The listing builds one solid part. Answer for the finished solid, in the listing's coordinates (mm). A direction names the side the tool comes from. Round coordinates to 2 decimals unless told otherwise and drop trailing zeros. Loops run counter-clockwise (first coordinate to the right, second up) from the corner with the lowest first, then second, coordinate; pieces in that order, holes last. Notation, with made-up numbers: M 82,42.25 L 119,42.25 A4 ccw 119,47.25 Z; hole C 84,42.5 d10. An arc over 180 degrees is marked long. Answer as a JSON object with one key per item and string values.
```python
from build123d import *

# Parameters (mm, degrees)
F0_W            = 25.4
F0_H            = 38.1
F1_DEPTH        = 12.7
F3_DEPTH        = 76.2
F4_W            = 25.4
F4_H            = 6.346226
F5_DEPTH        = 63.5
F7_DEPTH        = 25.4
F8_W            = 25.4
F8_H            = 6.35
F9_DEPTH        = 12.7
F11_DEPTH       = 25.4
F13_D           = 2.38125
F13_DEPTH       = 12.7
F13_CBORE_D     = 6.35
F13_CBORE_DEPTH = 3.175


with BuildPart() as f1:
    # F0 (on Front) → F1 (new body)
    with BuildSketch(Plane.XZ):
        with Locations((-20.66209, -15.939255)):
            Rectangle(F0_W, F0_H)
    extrude(amount=-F1_DEPTH)

    # F2 (on face) → F3 (join)
    with BuildSketch(Plane(origin=(0, 12.7, 0), x_dir=(-1, 0, 0), z_dir=(0, 1, 0))):
        Polygon((7.96209, -9.589255), (20.66209, -9.589255), (33.36209, -9.589255), (33.36209, 3.110745), (7.96209, 3.110745), align=None)
    extrude(amount=F3_DEPTH)

    # F4 (on face) → F5 (join)
    with BuildSketch(Plane(origin=(0, 0, -9.589255), x_dir=(1, 0, 0), z_dir=(0, 0, -1))):
        with Locations((-20.66209, -85.726887)):
            Rectangle(F4_W, F4_H)
    extrude(amount=F5_DEPTH)

    # F6 (on face) → F7 (join)
    with BuildSketch(Plane.YZ.offset(-7.96209)):
        Polygon((57.153774, -9.589255), (82.553774, -34.989255), (82.553774, -9.589255), align=None)
    extrude(amount=-F7_DEPTH)

    # F8 (on face) → F9 (join)
    with BuildSketch(Plane(origin=(0, 12.7, 0), x_dir=(-1, 0, 0), z_dir=(0, 1, 0))):
        with Locations((20.66209, -12.764255)):
            Rectangle(F8_W, F8_H)
    extrude(amount=F9_DEPTH)

    # F10 (on face) → F11 (cut, through all)
    with BuildSketch(Plane.YZ.offset(-7.96209)):
        Polygon((25.4, -15.939255), (25.4, -9.589255), (12.7, -15.939255), align=None)
    extrude(amount=-F11_DEPTH, mode=Mode.SUBTRACT)

    # F13
    with Locations(Plane(origin=(0, 12.7, 0), x_dir=(-1, 0, 0), z_dir=(0, 1, 0))):
        with Locations((20.66209, -25.464255)):
            CounterBoreHole(F13_D / 2, F13_CBORE_D / 2, F13_CBORE_DEPTH, depth=F13_DEPTH)


solid = f1.part
```
Item 1: Which of the six approach directions +Z, -Z, +X, -X, +Y, -Y give full straight-line access (tool end or side, diameter ignored) to faces 1 (the face through (-20, 41, -9.589)), 2 (the face through (-21, 82.554, -54)), 3 (the face through (-20.92, 4.696, -26.627))?
Values follow:
{"face 1": "-Z, +X, -X", "face 2": "-Z, +X, -X, -Y", "face 3": "-Y"}
Item 2: The part is cut by section D-D (y = 34). Give the vertices of the cut face in (x, z), then the cut area to 3 significant figures.
Values follow:
{"outline": "M -33.36,-9.59 L -7.96,-9.59 L -7.96,3.11 L -33.36,3.11 Z", "area": "323 mm^2"}
Item 3: The part is cut by section A-A (z = -14.5). Give the vertices of the cut face in (x, y), then the cut area to 3 significant figures.
Values follow:
{"outline": "M -33.36,0 L -7.96,0 L -7.96,15.58 L -33.36,15.58 Z; M -33.36,62.06 L -7.96,62.06 L -7.96,88.9 L -33.36,88.9 Z", "area": "1,080 mm^2"}
Item 4: The part is cut by section B-B (x = -12). Give the vertices of the cut face in (y, z).
Values follow:
{"outline": "M 0,-34.99 L 12.7,-34.99 L 12.7,-15.94 L 25.4,-9.59 L 57.15,-9.59 L 82.55,-34.99 L 82.55,-73.09 L 88.9,-73.09 L 88.9,3.11 L 0,3.11 Z"}
Item 5: The part is cut by section C-C (z = -67.5). Give the vertices of the cut face in (x, y), then the cut area to 3 significant figures.
Values follow:
{"outline": "M -33.36,82.55 L -7.96,82.55 L -7.96,88.9 L -33.36,88.9 Z", "area": "161 mm^2"}
Item 6: Straight lines are drawn through the part: line 1 (Y direction, x = -10.75, z = -46); line 2 (Y direction, x = -13, z = -17); line 3 (Y direction, x = -29.5, z = -13). For each, find the intervals that lie inside material, in ascending order.
Values follow:
{"line 1": "82.55 to 88.9", "line 2": "0 to 12.7, 64.56 to 88.9", "line 3": "0 to 18.58, 60.56 to 88.9"}
Item 7: Determine the mould class of faces 4 (the face through (-20.48, 19.14, -12.72)), 5 (the face through (-21, 44, 3.111)), 6 (the face through (-20.249, 11.135, -22.316)), 7 (the face through (-33.362, 48, -7)) for opening direction Z: released by +Z, released by -Z, zero draft, split by the parting line, or undercut.
Values follow:
{"face 4": "released by -Z", "face 5": "released by +Z", "face 6": "undercut", "face 7": "zero draft"}
Item 8: Flat-ended cylindrical pins translate along their axes: P1, Ø12.5, axis at x = -19, z = -61, coming from the -Y side; P2, Ø2, axis at x = -17, y = 45.5, coming from the -Z side; P3, Ø4, axis at x = -14.5, y = 7, coming from the -Z side; P4, Ø1.5, axis at x = -11, z = -27.5, coming from the -Y side. Find the tip coordinate at first contact, or state that the pin passes through.
Values follow:
{"P1": "y = 82.55", "P2": "z = -9.59", "P3": "z = -34.99", "P4": "y = 0"}
